from build123d import *

# Parameters (mm, degrees)
ESQUISSE1_W             = 32
ESQUISSE1_H             = 54
BOSS_EXTRU_1_DEPTH      = 8
ESQUISSE2_W             = 32
ESQUISSE2_H             = 4
BOSS_EXTRU_2_DEPTH      = 10
ESQUISSE3_W             = 8
ESQUISSE3_H             = 46
ENL_V_MAT_EXTRU_1_DEPTH = 9
ESQUISSE4_W             = 8
ESQUISSE4_H             = 46
ENL_V_MAT_EXTRU_2_DEPTH = 9
ESQUISSE5_R             = 2.5
ENL_V_MAT_EXTRU_3_DEPTH = 54
ESQUISSE6_W             = 14
ESQUISSE6_H             = 8
BOSS_EXTRU_3_DEPTH      = 14
ESQUISSE9_W             = 9
ESQUISSE9_H             = 10
ENL_V_MAT_EXTRU_6_DEPTH = 4
ESQUISSE10_W            = 14
ESQUISSE10_H            = 6
BOSS_EXTRU_4_DEPTH      = 7
ESQUISSE7_R             = 5
ENL_V_MAT_EXTRU_4_DEPTH = 55.118693403
ESQUISSE8_R             = 1.5
ENL_V_MAT_EXTRU_5_DEPTH = 7
ENL_V_MAT_EXTRU_7_DEPTH = 6
ESQUISSE12_W            = 14
ESQUISSE12_H            = 2
ENL_V_MAT_EXTRU_8_DEPTH = 66.299310869


with BuildPart() as part:
    # Esquisse1 → Boss.-Extru.1 (new body)
    with BuildSketch(Plane.XY):
        with Locations((16, 27)):
            Rectangle(ESQUISSE1_W, ESQUISSE1_H)
    extrude(amount=BOSS_EXTRU_1_DEPTH)

    # Esquisse2 → Boss.-Extru.2 (add)
    with BuildSketch(Plane.XY.offset(8)):
        with Locations((16, 52)):
            Rectangle(ESQUISSE2_W, ESQUISSE2_H)
    extrude(amount=BOSS_EXTRU_2_DEPTH)

    # Esquisse3 → Enlèv. mat.-Extru.1 (cut)
    with BuildSketch(Plane(origin=(32, 0, 0), x_dir=(0, 0, -1), z_dir=(1, 0, 0))):
        with Locations((-4, 27)):
            Rectangle(ESQUISSE3_W, ESQUISSE3_H)
    extrude(amount=-ENL_V_MAT_EXTRU_1_DEPTH, mode=Mode.SUBTRACT)

    # Esquisse4 → Enlèv. mat.-Extru.2 (cut)
    with BuildSketch(Plane.ZY):
        with Locations((4, 27)):
            Rectangle(ESQUISSE4_W, ESQUISSE4_H)
    extrude(amount=-ENL_V_MAT_EXTRU_2_DEPTH, mode=Mode.SUBTRACT)

    # Esquisse5 → Enlèv. mat.-Extru.3 (cut)
    with BuildSketch(Plane(origin=(0, 54, 0), x_dir=(1, 0, 0), z_dir=(0, 1, 0))):
        with Locations(Location((4, -4, 0), (0, 0, 270))):
            Circle(ESQUISSE5_R)
        with Locations(Location((28, -4, 0), (0, 0, 270))):
            Circle(ESQUISSE5_R)
    extrude(amount=-ENL_V_MAT_EXTRU_3_DEPTH, mode=Mode.SUBTRACT)

    # Esquisse6 → Boss.-Extru.3 (add)
    with BuildSketch(Plane(origin=(0, 0, 0), x_dir=(-1, 0, 0), z_dir=(0, 0, -1))):
        with Locations((-16, 10.240309664)):
            Rectangle(ESQUISSE6_W, ESQUISSE6_H)
    extrude(amount=BOSS_EXTRU_3_DEPTH)

    # Esquisse9 → Enlèv. mat.-Extru.6 (cut)
    with BuildSketch(Plane(origin=(0, 54, 0), x_dir=(1, 0, 0), z_dir=(0, 1, 0))):
        with Locations((27.5, -13)):
            Rectangle(ESQUISSE9_W, ESQUISSE9_H)
        with Locations((4.5, -13)):
            Rectangle(ESQUISSE9_W, ESQUISSE9_H)
    extrude(amount=-ENL_V_MAT_EXTRU_6_DEPTH, mode=Mode.SUBTRACT)

    # Esquisse10 → Boss.-Extru.4 (add)
    with BuildSketch(Plane(origin=(0, 0, 0), x_dir=(-1, 0, 0), z_dir=(0, 0, -1))):
        with Locations((-16, 39.240309664)):
            Rectangle(ESQUISSE10_W, ESQUISSE10_H)
    extrude(amount=BOSS_EXTRU_4_DEPTH)

    # Esquisse7 → Enlèv. mat.-Extru.4 (cut, through all)
    with BuildSketch(Plane(origin=(0, 14.240309664, 0), x_dir=(1, 0, 0), z_dir=(0, 1, 0))):
        with Locations(Location((16, 7, 0), (0, 0, 270))):
            Circle(ESQUISSE7_R)
    extrude(amount=-ENL_V_MAT_EXTRU_4_DEPTH, mode=Mode.SUBTRACT)

    # Esquisse8 → Enlèv. mat.-Extru.5 (cut)
    with BuildSketch(Plane(origin=(0, 0, -14), x_dir=(-1, 0, 0), z_dir=(0, 0, -1))):
        with Locations((-16, 10.240309664)):
            Circle(ESQUISSE8_R)
    extrude(amount=-ENL_V_MAT_EXTRU_5_DEPTH, mode=Mode.SUBTRACT)

    # Esquisse11 → Enlèv. mat.-Extru.7 (cut)
    with BuildSketch(Plane(origin=(0, 42.240309664, 0), x_dir=(1, 0, 0), z_dir=(0, 1, 0))):
        Polygon((21, 7), (16, 2), (11, 7), align=None)
    extrude(amount=-ENL_V_MAT_EXTRU_7_DEPTH, mode=Mode.SUBTRACT)

    # Esquisse12 → Enlèv. mat.-Extru.8 (cut, through all)
    with BuildSketch(Plane(origin=(0, 54, 0), x_dir=(1, 0, 0), z_dir=(0, 1, 0))):
        with Locations((16, -17)):
            Rectangle(ESQUISSE12_W, ESQUISSE12_H)
    extrude(amount=-ENL_V_MAT_EXTRU_8_DEPTH, mode=Mode.SUBTRACT)


solid = part.part
Part model, mm, in its own coordinate system. A direction names the side the tool comes from. Coordinates: 2 decimals unless noted, no trailing zeros. Loops run counter-clockwise (first coordinate to the right, second up) from the corner with the lowest first, then second, coordinate; pieces in that order, holes last. Notation, with made-up numbers: (-6.5, 5.5) -> (34.5, 5.5) arc R14 ccw to (34.5, 21.5) -> close; hole circle Ø1 at (65.25, 68.5). An arc over 180 degrees is marked (long way). Use a Markdown table: item, result. Add a question column.
Item 1: Band-saw the part on B-B on z = 4. Write the cut outline in (x, y), plus the area to 3 significant figures.
Item 2: Band-saw the part on C-C on x = 28. Write the cut outline in (y, z).
Item 3: Band-saw the part on A-A on x = 19. Write the cut outline in (y, z), plus the area to 3 significant figures.
Item 4: Flat gauge pins, fed straight in: P1, Ø6, axis at x = 4, z = 4, coming from the +Y side; P2, Ø11, axis at x = 14, z = -8, coming from the +Y side; P3, Ø1.6, axis at x = 10.5, y = 40, coming from the -Z side; P4, Ø2, axis at x = 27.5, y = 52, coming from the +Z side. Where does each tip first touch, or does it go through?
Item 5: Probe probe 1 along X at (y, z) = (52, 4); probe 2 along Y at (x, z) = (16, -13); probe 3 along X at (y, z) = (9.25, -7). List the from-to ranges inside material, lowest first.
Item 6: Band-saw the part on D-D on y = 13. Write the cut outline in (x, z).
Item 7: Which spindle directions (+Z, -Z, +X, -X, +Y, -Y) get a long thin tool onto all of the face, cutting with end or side? Do faces 1 (the flat face through (23, 52, 12)), 2 (the flat face through (16, 50, 0)), 3 (the flat face through (9, 52, 12)), 4 (the flat face through (14, 39, -4)). Say none if no direction does.
Item 8: Pull direction Y, two halves, no side cores. Call faces 5 (the flat face through (18, 14.24, -2)), 6 (the flat face through (32, 52, 4)), 7 (the flat face through (16, 50, 12)): +Y half, -Y half, draft (parallel to the pull), parting line (faces both ways), or undercut.
Geometry says:
| question | item | result |
|---|---|---|
| 1 | outline | (0, 0) -> (1.5, 0) -> (1.5, 4) -> (0, 4) -> close; (0, 50) -> (1.5, 50) -> (1.5, 54) -> (0, 54) -> close; (6.5, 0) -> (25.5, 0) -> (25.5, 4) -> (23, 4) -> (23, 50) -> (25.5, 50) -> (25.5, 54) -> (6.5, 54) -> (6.5, 50) -> (9, 50) -> (9, 4) -> (6.5, 4) -> close; (30.5, 0) -> (32, 0) -> (32, 4) -> (30.5, 4) -> close; (30.5, 50) -> (32, 50) -> (32, 54) -> (30.5, 54) -> close |
| 1 | area | 820 mm² |
| 2 | outline | (0, 0) -> (4, 0) -> (4, 1.5) -> (0, 1.5) -> close; (0, 6.5) -> (4, 6.5) -> (4, 8) -> (0, 8) -> close; (50, 0) -> (54, 0) -> (54, 1.5) -> (50, 1.5) -> close; (50, 6.5) -> (54, 6.5) -> (54, 8) -> (50, 8) -> close |
| 3 | outline | (0, 0) -> (6.24, 0) -> (6.24, -3) -> (14.24, -3) -> (14.24, 0) -> (36.24, 0) -> (36.24, -5) -> (42.24, -5) -> (42.24, 0) -> (54, 0) -> (54, 16) -> (50, 16) -> (50, 8) -> (0, 8) -> close; (6.24, -14) -> (14.24, -14) -> (14.24, -11) -> (6.24, -11) -> close |
| 3 | area | 542 mm² |
| 4 | P1 | y = 54 |
| 4 | P2 | y = 42.24 |
| 4 | P3 | z = -7 |
| 4 | P4 | z = 8 |
| 5 | probe 1 | 0 to 1.5, 6.5 to 25.5, 30.5 to 32 |
| 5 | probe 2 | 6.24 to 8.74, 11.74 to 14.24 |
| 5 | probe 3 | 9 to 11, 21 to 23 |
| 6 | outline | (9, -14) -> (23, -14) -> (23, 8) -> (9, 8) -> close; hole circle Ø10 at (16, -7) |
| 7 | face 1 | +Z, +X, +Y, -Y |
| 7 | face 2 | -Z, +X, -X, +Y |
| 7 | face 3 | +Z, -X, +Y, -Y |
| 7 | face 4 | -Z, +Y, -Y |
| 8 | face 5 | undercut |
| 8 | face 6 | draft |
| 8 | face 7 | -Y half |
